```python
from build123d import *

# Parameters (mm, degrees)
F1_ANGLE = 68


# Not quite as in the source:
# - a feature of the source that left no trace in its solid (it failed there, or was rolled back) is left out


with BuildPart() as f1:
    # F0 (on Front) → F1 (revolve)
    with BuildSketch(Plane.XZ):
        with BuildLine():
            Line((-15.24, 0), (0, 0))
            Line((0, 0), (0, 50.8))
            Line((0, 50.8), (-6.35, 50.8))
            Line((-6.35, 50.8), (-4.7617064118, 41.792339449))
            ThreePointArc((-4.7617064118, 41.792339449), (-4.8311637627, 41.5331210865), (-5.0743828734, 41.4197061526))
            Line((-5.0743828734, 41.4197061526), (-6.2835011077, 41.4197061526))
            ThreePointArc((-6.2835011077, 41.4197061526), (-6.5080075107, 41.3267125556), (-6.6010011077, 41.1022061526))
            Line((-6.6010011077, 41.1022061526), (-6.6010011077, 40.4672061526))
            ThreePointArc((-6.6010011077, 40.4672061526), (-6.5080075107, 40.2426997495), (-6.2835011077, 40.1497061526))
            Line((-6.2835011077, 40.1497061526), (-5.0743828734, 40.1497061526))
            ThreePointArc((-5.0743828734, 40.1497061526), (-4.8311637627, 40.0362912186), (-4.7617064118, 39.7770728561))
            Line((-4.7617064118, 39.7770728561), (-5.2010717431, 37.2853082403))
            ThreePointArc((-5.2010717431, 37.2853082403), (-5.3096631386, 37.0972224261), (-5.5137482047, 37.0229415367))
            Line((-5.5137482047, 37.0229415367), (-6.8348340718, 37.0229415367))
            ThreePointArc((-6.8348340718, 37.0229415367), (-7.0593404748, 36.9299479398), (-7.1523340718, 36.7054415367))
            Line((-7.1523340718, 36.7054415367), (-7.1523340718, 36.0704415367))
            ThreePointArc((-7.1523340718, 36.0704415367), (-7.2453276688, 35.8459351337), (-7.4698340718, 35.7529415367))
            Line((-7.4698340718, 35.7529415367), (-8.7398340718, 35.7529415367))
            ThreePointArc((-8.7398340718, 35.7529415367), (-8.9643404748, 35.6599479398), (-9.0573340718, 35.4354415367))
            Line((-9.0573340718, 35.4354415367), (-9.0573340718, 34.8004415367))
            ThreePointArc((-9.0573340718, 34.8004415367), (-8.9643404748, 34.5759351337), (-8.7398340718, 34.4829415367))
            Line((-8.7398340718, 34.4829415367), (-3.5686493249, 34.4829415367))
            ThreePointArc((-3.5686493249, 34.4829415367), (-3.3254302142, 34.3695266028), (-3.2559728633, 34.1103082403))
            Line((-3.2559728633, 34.1103082403), (-7.113602572, 12.2326030065))
            ThreePointArc((-7.113602572, 12.2326030065), (-7.2221939675, 12.0445171922), (-7.4262790336, 11.9702363029))
            Line((-7.4262790336, 11.9702363029), (-8.1123649007, 11.9702363029))
            ThreePointArc((-8.1123649007, 11.9702363029), (-8.3368713037, 11.8772427059), (-8.4298649007, 11.6527363029))
            Line((-8.4298649007, 11.6527363029), (-8.4298649007, 8.9432889844))
            ThreePointArc((-8.4298649007, 8.9432889844), (-8.4596121783, 8.8091076862), (-8.5432798346, 8.7000698737))
            Line((-8.5432798346, 8.7000698737), (-15.1265850661, 3.176020882))
            ThreePointArc((-15.1265850661, 3.176020882), (-15.2102527224, 3.0669830694), (-15.24, 2.9328017713))
            Line((-15.24, 2.9328017713), (-15.24, 0))
        make_face()
    revolve(axis=Axis((0, 0, 25.4), (0, 0, 1)), revolution_arc=F1_ANGLE)


solid = f1.part
```
The model under review builds one solid part; all positions refer to its coordinate system, in mm. A direction names the side the tool comes from. Give positions to 0.01 mm unless a question says otherwise; leave off trailing zeros. Write each loop counter-clockwise with the first axis right and the second up, starting at its lowest first coordinate (ties: lowest second). Pieces come first, ordered by that corner, then holes. Notation, with made-up numbers: M 52.5,40.25 L 98.5,40.25 A18 ccw 98.5,74.25 Z; hole C -23.5,52.25 d6. An arc over 180 degrees is marked long. Write item = value, one per line. Start each with the question number.
Q1. We need section A-A (z = 45). State the section outline as (x, y) points, plus the area to 3 significant figures.
Q2. Mouldability with a two-part tool opening along Z and no side actions: class faces 1 (the face through (-3, -2, 50.8)), 2 (the face through (-5, -3, 37.023)), 3 (the face through (-12.705, -8.417, 1.446)) as released by +Z, released by -Z, zero draft, split by the parting line, or undercut.
Q3. For line 1 (X direction, y = -2.5, z = 43); line 2 (Z direction, x = -9, y = -9); line 3 (Y direction, x = -5, z = 10), list the stretches that pass through material, from the lowest coordinate up.
Q4. We need section B-B (z = 28.5). State the section outline as (x, y) points.
Q5. Machinability: for faces 4 (the face through (-6.443, -4.071, 35.753)), 5 (the face through (-4.4, -3.1, 41.42)), 6 (the face through (-4, 0, 20)), which of the approach directions +Z, -Z, +X, -X, +Y, -Y give a long, thin tool a straight path to every point of the face, cutting with its end or side? Answer none if there is none.
Q6. Clearance check with flat-ended pins moving along their axes: pin 1 (2 mm diameter, centred on x = -6.5, y = -4, fed in from +Z); pin 2 (2 mm diameter, centred on x = -13, y = -5.5, fed in from +Z); pin 3 (1 mm diameter, centred on x = -3.5, z = 38.5, fed in from -Y); pin 4 (1 mm diameter, centred on x = -11.5, y = -11, fed in from +Z). State where each tip first meets the part, or that it passes through.
Result set:
q1.outline = M -5.33,0 A5.33 ccw -2,-4.94 L 0,0 Z
q1.area = 16.8 mm2
q2.face_1 = released by +Z
q2.face_2 = undercut
q2.face_3 = zero draft
q3.line_1 = -4.3 to -1.01
q3.line_2 = 0 to 5.19
q3.line_3 = -6.79 to 0
q4.outline = M -4.25,0 A4.25 ccw -1.59,-3.94 L 0,0 Z
q5.face_4 = +Z, -X, -Y
q5.face_5 = -X, -Y
q5.face_6 = +Z, -Z, +X, -X, +Y
q6.pin_1 = 37.02
q6.pin_2 = 4.86
q6.pin_3 = -4
q6.pin_4 = through
